```python
from build123d import *

# Parameters (mm, degrees)
SKETCH1_R           = 19.05
SKETCH1_R_2         = 13.97
BOSS_EXTRUDE1_DEPTH = 30.48
SKETCH2_R           = 13.97
BOSS_EXTRUDE2_DEPTH = 6.35
SKETCH7_R           = 5.08
CUT_EXTRUDE4_DEPTH  = 7.35
SKETCH9_R           = 7.62
SKETCH9_R_2         = 5.08
BOSS_EXTRUDE3_DEPTH = 13.97
SKETCH10_R          = 7.62
SKETCH10_R_2        = 3.81
BOSS_EXTRUDE4_DEPTH = 7.62
FILLET1_R           = 2.54


with BuildPart() as part:
    # Sketch1 → Boss-Extrude1 (new body)
    with BuildSketch(Plane(origin=(0, 0, 0), x_dir=(1, 0, 0), z_dir=(0, 1, 0))):
        Circle(SKETCH1_R)
        Circle(SKETCH1_R_2, mode=Mode.SUBTRACT)
    extrude(amount=BOSS_EXTRUDE1_DEPTH)

    # Sketch2 → Boss-Extrude2 (add)
    with BuildSketch(Plane.XZ):
        Circle(SKETCH2_R)
    extrude(amount=-BOSS_EXTRUDE2_DEPTH)

    # Sketch7 → Cut-Extrude4 (cut, through all)
    with BuildSketch(Plane(origin=(0, 6.35, 0), x_dir=(1, 0, 0), z_dir=(0, 1, 0))):
        Circle(SKETCH7_R)
    extrude(amount=-CUT_EXTRUDE4_DEPTH, mode=Mode.SUBTRACT)

    # Sketch9 → Boss-Extrude3 (add)
    with BuildSketch(Plane(origin=(0, 6.35, 0), x_dir=(1, 0, 0), z_dir=(0, 1, 0))):
        Circle(SKETCH9_R)
        Circle(SKETCH9_R_2, mode=Mode.SUBTRACT)
    extrude(amount=BOSS_EXTRUDE3_DEPTH)

    # Sketch10 → Boss-Extrude4 (add)
    with BuildSketch(Plane(origin=(0, 20.32, 0), x_dir=(1, 0, 0), z_dir=(0, 1, 0))):
        Circle(SKETCH10_R)
        Circle(SKETCH10_R_2, mode=Mode.SUBTRACT)
    extrude(amount=BOSS_EXTRUDE4_DEPTH)

    # Fillet1
    fillet1_edges = [part.edges().sort_by_distance(p)[0] for p in [
        (-3.81, 27.94, 0),
    ]]
    fillet(fillet1_edges, radius=FILLET1_R)


solid = part.part
```
Geometry check sheet. Reference: the model listing, model coordinates, mm. A direction names the side the tool comes from. Give positions to 0.01 mm unless a question says otherwise; leave off trailing zeros. Order: outer loops, then holes, each group sorted by start corner. A loop starts at its lowest first (then second) coordinate and runs counter-clockwise, first axis right, second up.
1. Gauge pin test, flat ends, axial feed: pin 1 Ø14 at (x, z) = (-2.5, -4) entering from +Y; pin 2 Ø5 at (x, y) = (14.5, 10.5) entering from +Z; pin 3 Ø3 at (x, y) = (11, 10) entering from +Z. Record the tip position at first contact, or that the pin passes through.
2. Section check A-A, the plane x = 0. Enter the section's corners in (y, z), and give its area (3 significant figures).
3. Section check C-C, the plane y = 18. Enter the section's corners in (x, z), and give its area (3 significant figures).
4. Section check B-B, the plane z = 0. Enter the section's corners in (x, y).
5. Access from +Z, -Z, +X, -X, +Y, -Y to the whole of each face (thin tool, end or side, straight path). Record for faces 4 (the face through (-3, 27.94, -6)), 5 (the face through (-0.83, 22.82, 3.72)).
6. Section check D-D, the plane y = 5. Enter the section's corners in (x, z), and give its area (3 significant figures).
7. Release check for a two-part mould opening along Z. For faces 1 (the face through (1, 20.32, -4)), 2 (the face through (-15.12, 15.03, 11.59)), 3 (the face through (4, 0, -4)) record: pulls with the +Z half, pulls with the -Z half, needs draft (parallel to the pull), parting line crosses it, or undercut.
8. Thickness scan on L1, parallel to Z at x = 0, y = 21; L2, parallel to Z at x = 0, y = 14.75. Record the ranges inside material, lowest first.
Values follow:
1. pin 1: stops at y = 27.94
1. pin 2: stops at z = 14.8
1. pin 3: stops at z = 16.51
2. outline: (0, -19.05) - (30.48, -19.05) - (30.48, -13.97) - (6.35, -13.97) - (6.35, -7.62) - (27.94, -7.62) - (27.94, -6.35) arc R2.54 ccw to (25.4, -3.81) - (20.32, -3.81) - (20.32, -5.08) - (0, -5.08) - close; (0, 5.08) - (20.32, 5.08) - (20.32, 3.81) - (25.4, 3.81) arc R2.54 ccw to (27.94, 6.35) - (27.94, 7.62) - (6.35, 7.62) - (6.35, 13.97) - (30.48, 13.97) - (30.48, 19.05) - (0, 19.05) - close
2. area: 549 mm2
3. outline: circle Ø38.1 at (0, 0); circle Ø15.24 at (0, 0); hole circle Ø27.94 at (0, 0); hole circle Ø10.16 at (0, 0)
3. area: 628 mm2
4. outline: (-19.05, 0) - (-5.08, 0) - (-5.08, 20.32) - (-3.81, 20.32) - (-3.81, 25.4) arc R2.54 ccw to (-6.35, 27.94) - (-7.62, 27.94) - (-7.62, 6.35) - (-13.97, 6.35) - (-13.97, 30.48) - (-19.05, 30.48) - close; (3.81, 20.32) - (5.08, 20.32) - (5.08, 0) - (19.05, 0) - (19.05, 30.48) - (13.97, 30.48) - (13.97, 6.35) - (7.62, 6.35) - (7.62, 27.94) - (6.35, 27.94) arc R2.54 ccw to (3.81, 25.4) - close
5. face 4: +Y
5. face 5: +Y, -Y
6. outline: circle Ø38.1 at (0, 0); hole circle Ø10.16 at (0, 0)
6. area: 1,060 mm2
7. face 1: undercut
7. face 2: parting line crosses it
7. face 3: needs draft
8. L1: z = -19.05 to -13.97, -7.62 to -3.81, 3.81 to 7.62, 13.97 to 19.05
8. L2: z = -19.05 to -13.97, -7.62 to -5.08, 5.08 to 7.62, 13.97 to 19.05
